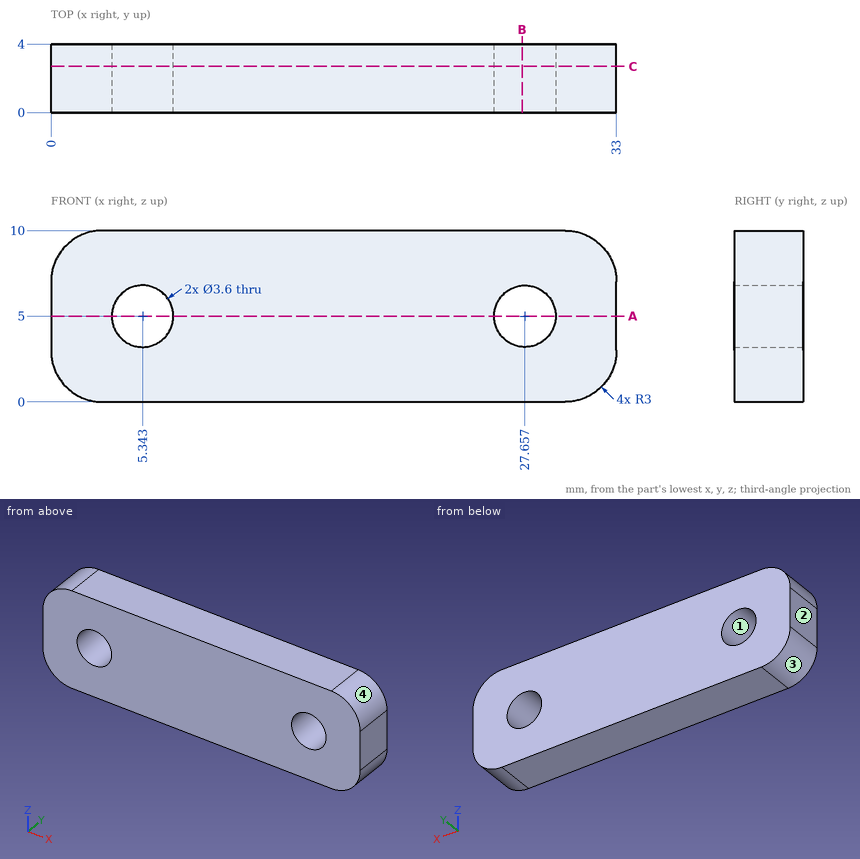
Input: dimensioned drawing with shaded views. Units: mm. Origin: part minimum x, y, z. Round coordinates to 2 decimals unless told otherwise and drop trailing zeros. Order: outer loops, then holes, each group sorted by start corner. A loop starts at its lowest first (then second) coordinate and runs counter-clockwise, first axis right, second up. Notation, with made-up numbers: (78, 42.25) - (92, 42.25) arc R14 cw to (92, 56.25) - close; hole circle Ø4 at (-16.5, 39.5). An arc over 180 degrees is marked (long way). Write item = value, one per line. Start each with the question number.
Q1. Pull-direction query (Z, two-part tool) for the marked faces 1, 2, 3 and 4; classes: +Z half, -Z half, draft (parallel to the pull), parting line (faces both ways), or undercut.
Q2. Cut plane A-A on z = 5. Return the cut outline in (x, y).
Q3. Pin query (flat end, axial travel): pin 1 (4 mm diameter, centred on x = 5.343, z = 5, fed in from +Y); pin 2 (2 mm diameter, centred on x = 27.657, z = 5, fed in from -Y). Return the tip coordinate at first contact, or that it passes through.
Q4. Cut plane C-C on y = 2.7. Return the cut outline in (x, z), and give its area (3 significant figures).
Q5. Ray query, line 1 (X direction, y = 3.1, z = 5); line 2 (X direction, y = 2.75, z = 5.75); line 3 (Z direction, x = 4.5, y = 0.8). Return the intervals inside material, ascending. Write a range as from..to.
Q6. Cut plane B-B on x = 27.5. Return the cut outline in (y, z).
Outcome:
q1.face_1 = undercut
q1.face_2 = draft
q1.face_3 = -Z half
q1.face_4 = +Z half
q2.outline = (0, 0) - (3.54, 0) - (3.54, 4) - (0, 4) - close; (7.14, 0) - (25.86, 0) - (25.86, 4) - (7.14, 4) - close; (29.46, 0) - (33, 0) - (33, 4) - (29.46, 4) - close
q3.pin_1 = 4
q3.pin_2 = through
q4.outline = (0, 3) arc R3 ccw to (3, 0) - (30, 0) arc R3 ccw to (33, 3) - (33, 7) arc R3 ccw to (30, 10) - (3, 10) arc R3 ccw to (0, 7) - close; hole circle Ø3.6 at (5.34, 5); hole circle Ø3.6 at (27.66, 5)
q4.area = 302 mm^2
q5.line_1 = 0..3.54, 7.14..25.86, 29.46..33
q5.line_2 = 0..3.71, 6.98..26.02, 29.29..33
q5.line_3 = 0..3.41, 6.59..10
q6.outline = (0, 0) - (4, 0) - (4, 3.21) - (0, 3.21) - close; (0, 6.79) - (4, 6.79) - (4, 10) - (0, 10) - close
